Here's how the part is built. I have some questions about the finished solid (model axes, mm). Coordinates: 2 decimals unless noted, no trailing zeros. Loops run counter-clockwise (first coordinate to the right, second up) from the corner with the lowest first, then second, coordinate; pieces in that order, holes last. Notation, with made-up numbers: (8.25, 31) - (30.25, 31) arc R22 cw to (30.25, 54) - close; hole circle Ø1 at (14, -22.5). An arc over 180 degrees is marked (long way). Use a Markdown table: item, result.
```python
from build123d import *

# Parameters (mm, degrees)
F1_DEPTH = 100


with BuildPart() as f1:
    # F0 (on Front) → F1 (new body)
    with BuildSketch(Plane.XZ):
        Polygon((0, 20), (0, 0), (50, 0), (50, 10), (50, 20), align=None)
        Polygon((50, 20), (50, 10), (100, 10), align=None)
        Polygon((50, 10), (50, 0), (100, 10), align=None)
    extrude(amount=F1_DEPTH)


solid = f1.part
```
Q1. I want a section at C-C, the plane z = 1.5. Write out the boundary of the cut face in (x, y), then the cut area to 3 significant figures.
Check values:
| item | result |
|---|---|
| outline | (0, -100) - (57.5, -100) - (57.5, 0) - (0, 0) - close |
| area | 5,750 mm^2 |
Q2. Please list where these lines run through material, in increasing order: L1, parallel to Z at x = 67, y = -5; L2, parallel to Z at x = 90.5, y = -94.5. Write a range as from..to.
Check values:
| item | result |
|---|---|
| L1 | 3.4..16.6 |
| L2 | 8.1..11.9 |
Q3. I want a section at A-A, the plane y = -57. Write out the boundary of the cut face in (x, z), then the cut area to 3 significant figures.
Check values:
| item | result |
|---|---|
| outline | (0, 0) - (50, 0) - (100, 10) - (50, 20) - (0, 20) - close |
| area | 1,500 mm^2 |
Q4. Will these pins go through, and if not, where does the flat tip stop? P1, Ø1, axis at x = 58, y = -24.5, coming from the -Z side; P2, Ø4, axis at x = 68.5, y = -83, coming from the +Z side; P3, Ø6, axis at x = 79.5, y = -39, coming from the -Z side; P4, Ø3, axis at x = 24.5, z = 7, coming from the +Y side.
Check values:
| item | result |
|---|---|
| P1 | z = 1.5 |
| P2 | z = 16.7 |
| P3 | z = 5.3 |
| P4 | y = 0 |
Q5. I want a section at B-B, the plane x = 85.5. Write out the boundary of the cut face in (y, z), then the cut area to 3 significant figures.
Check values:
| item | result |
|---|---|
| outline | (-100, 7.1) - (0, 7.1) - (0, 12.9) - (-100, 12.9) - close |
| area | 580 mm^2 |
